```python
from build123d import *

# Parameters (mm, degrees)
SKETCH1_R             = 1.5875
SKETCH1_R_2           = 2.1844
BOSS_EXTRUDE2_DEPTH   = 1.524
BOSS_EXTRUDE3_DEPTH   = 15.875
SKETCH3_R             = 2.1844
BOSS_EXTRUDE4_DEPTH   = 1.778
BOSS_EXTRUDE4_2_DEPTH = 1.778
CUT_EXTRUDE1_DEPTH    = 9.398
SKETCH6_R             = 2.1844
BOSS_EXTRUDE5_DEPTH   = 16.256


with BuildPart() as part:
    # Sketch1 → Boss-Extrude2 (new body)
    with BuildSketch(Plane(origin=(0, 0, 0), x_dir=(1, 0, 0), z_dir=(0, 1, 0))):
        with BuildLine():
            Line((-50.746188486, 35.427401309), (-17.726188486, 35.427401309))
            ThreePointArc((-17.726188486, 35.427401309), (-16.828162874, 35.055426921), (-16.456188486, 34.157401309))
            Line((-16.456188486, 34.157401309), (-16.456188486, 27.108901309))
            ThreePointArc((-16.456188486, 27.108901309), (-16.084214098, 26.210875697), (-15.186188486, 25.838901309))
            Line((-15.186188486, 25.838901309), (-1.470188486, 25.838901309))
            ThreePointArc((-1.470188486, 25.838901309), (-0.572162874, 25.466926921), (-0.200188486, 24.568901309))
            Line((-0.200188486, 24.568901309), (-0.200188486, 10.725901309))
            ThreePointArc((-0.200188486, 10.725901309), (-0.572162874, 9.827875697), (-1.470188486, 9.455901309))
            Line((-1.470188486, 9.455901309), (-15.186188486, 9.455901309))
            ThreePointArc((-15.186188486, 9.455901309), (-16.084214098, 9.083926921), (-16.456188486, 8.185901309))
            Line((-16.456188486, 8.185901309), (-16.456188486, 1.137401309))
            ThreePointArc((-16.456188486, 1.137401309), (-16.828162874, 0.239375697), (-17.726188486, -0.132598691))
            Line((-17.726188486, -0.132598691), (-50.746188486, -0.132598691))
            ThreePointArc((-50.746188486, -0.132598691), (-51.644214098, 0.239375697), (-52.016188486, 1.137401309))
            Line((-52.016188486, 1.137401309), (-52.016188486, 34.157401309))
            ThreePointArc((-52.016188486, 34.157401309), (-51.644214098, 35.055426921), (-50.746188486, 35.427401309))
        make_face()
        with Locations(Location((-49.539688486, 32.900101309, 0), (0, 0, 90))):
            Circle(SKETCH1_R, mode=Mode.SUBTRACT)
        with Locations(Location((-18.907288486, 32.900101309, 0), (0, 0, 90))):
            Circle(SKETCH1_R, mode=Mode.SUBTRACT)
        with Locations(Location((-18.907288486, 2.394701309, 0), (0, 0, 90))):
            Circle(SKETCH1_R, mode=Mode.SUBTRACT)
        with Locations(Location((-49.539688486, 2.394701309, 0), (0, 0, 90))):
            Circle(SKETCH1_R, mode=Mode.SUBTRACT)
        with Locations(Location((-4.111788486, 21.165301309, 0), (0, 0, 90))):
            Circle(SKETCH1_R_2, mode=Mode.SUBTRACT)
        with Locations(Location((-4.111788486, 14.129501309, 0), (0, 0, 90))):
            Circle(SKETCH1_R_2, mode=Mode.SUBTRACT)
    extrude(amount=BOSS_EXTRUDE2_DEPTH)

    # Sketch2 → Boss-Extrude3 (add)
    with BuildSketch(Plane(origin=(0, 1.524, 0), x_dir=(1, 0, 0), z_dir=(0, 1, 0))):
        with BuildLine():
            Line((-0.249338446, 12.681643767), (-2.605441809, 10.307979525))
            ThreePointArc((-2.605441809, 10.307979525), (-2.77070914, 10.196884511), (-2.96598326, 10.157853612))
            Line((-2.96598326, 10.157853612), (-5.158955649, 10.157853612))
            ThreePointArc((-5.158955649, 10.157853612), (-5.354367589, 10.196941921), (-5.519707394, 10.308191511))
            Line((-5.519707394, 10.308191511), (-7.872832313, 12.681643767))
            Line((-7.872832313, 12.681643767), (-7.872832313, 24.873643767))
            ThreePointArc((-7.872832313, 24.873643767), (-7.724042558, 25.232854011), (-7.364832313, 25.381643767))
            Line((-7.364832313, 25.381643767), (-0.757338446, 25.381643767))
            ThreePointArc((-0.757338446, 25.381643767), (-0.398128202, 25.232854011), (-0.249338446, 24.873643767))
            Line((-0.249338446, 24.873643767), (-0.249338446, 12.681643767))
        make_face()
    extrude(amount=BOSS_EXTRUDE3_DEPTH)

    # Sketch4 → Cut-Extrude1 (cut)
    with BuildSketch(Plane(origin=(0, 17.399, 0), x_dir=(1, 0, 0), z_dir=(0, 1, 0))):
        Polygon((-7.237832313, 24.873643767), (-7.237832313, 12.681643767), (-5.158955649, 10.792853612), (-2.96598326, 10.792853612), (-0.884338446, 12.681643767), (-0.884338446, 24.873643767), align=None)
    extrude(amount=-CUT_EXTRUDE1_DEPTH, mode=Mode.SUBTRACT)



with BuildPart() as body_2:
    # Sketch3 → Boss-Extrude4 (new body)
    with BuildSketch(Plane.XZ):
        with Locations(Location((-4.111788486, -14.129501309, 0), (0, 0, 270))):
            Circle(SKETCH3_R)
    extrude(amount=BOSS_EXTRUDE4_DEPTH)


with BuildPart() as body_3:
    # Sketch3 → Boss-Extrude4 2 (new body)
    with BuildSketch(Plane.XZ):
        with Locations(Location((-4.111788486, -21.165301309, 0), (0, 0, 270))):
            Circle(SKETCH3_R)
    extrude(amount=BOSS_EXTRUDE4_2_DEPTH)


with BuildPart() as part_1:
    add(part.part)

    add(body_2.part)  # Boss-Extrude5 merges body 2

    add(body_3.part)  # Boss-Extrude5 merges body 3
    # Sketch6 → Boss-Extrude5 (add)
    with BuildSketch(Plane.XZ):
        with Locations(Location((-4.111788486, -14.129501309, 0), (0, 0, 90))):
            Circle(SKETCH6_R)
        with Locations(Location((-4.111788486, -21.165301309, 0), (0, 0, 270))):
            Circle(SKETCH6_R)
    extrude(amount=-BOSS_EXTRUDE5_DEPTH)


solid = part_1.part
```
Could you check a few things on this model? Use its own coordinates, in mm. A direction names the side the tool comes from. Coordinates: 2 decimals unless noted, no trailing zeros. Write each loop counter-clockwise with the first axis right and the second up, starting at its lowest first coordinate (ties: lowest second). Pieces come first, ordered by that corner, then holes. Notation, with made-up numbers: (19.25, -9) -> (71.25, -9) arc R17 ccw to (71.25, 11) -> close; hole circle Ø4 at (4.25, -8.75). An arc over 180 degrees is marked (long way). One line per question, with ' | ' between items. Start each with the question number.
1. If we section it at C-C (y = 3.5): Please give me the cut outline in (x, z), and give its area (3 significant figures).
2. For faces 5 (the face through (-1.41, 9.35, -11.51)), 6 (the face through (-16.456, 1, -31)), 7 (the face through (-5.4, -0.9, -19.4)), 8 (the face through (-0.249, 9, -19)), 9 (the face through (-4, 16.256, -14)), which set-ups out of +Z, -Z, +X, -X, +Y, -Y let a thin tool reach every point of the face, with its end or its side?
3. Please list where these lines run through material, in increasing order: line 1 along X through (y, z) = (9, -14); line 2 along X through (y, z) = (8.5, -24); line 3 along X through (y, z) = (14, -16).
4. Will these pins go through, and if not, where does the flat tip stop? P1, Ø1.7, axis at x = -6.5, y = 0.5, coming from the +Z side; P2, Ø12, axis at x = -13, z = -26, coming from the -Y side; P3, Ø10, axis at x = -42, z = -27.5, coming from the +Y side.
5. If we section it at D-D (x = -25): Please give me the cut outline in (y, z).
6. Thinking about a two-plate mould opening in Z: for faces 1 (the face through (-4, 9, -25.382)), 2 (the face through (-4, 13, -24.874)), 3 (the face through (-4, -1.778, -21)), 4 (the face through (-50.61, 0.75, -1.22)), which applies, pulls with the +Z half, pulls with the -Z half, needs draft (parallel to the pull), parting line crosses it, or undercut?
7. If we section it at B-B (y = 11.25): Please give me the cut outline in (x, z), and give its area (3 significant figures).
8. If we section it at A-A (z = -17.5): Please give me the cut outline in (x, y).
Return value:
1) outline: (-7.87, -24.87) arc R0.51 ccw to (-7.36, -25.38) -> (-0.76, -25.38) arc R0.51 ccw to (-0.25, -24.87) -> (-0.25, -12.68) -> (-2.61, -10.31) arc R0.51 ccw to (-2.97, -10.16) -> (-5.16, -10.16) arc R0.51 ccw to (-5.52, -10.31) -> (-7.87, -12.68) -> close | area: 110 mm²
2) face 5: +Z, +X, +Y | face 6: -Z, +X, +Y, -Y | face 7: -Y | face 8: +Z, -Z, +X, +Y | face 9: +Y
3) line 1: x = -7.87 to -7.24, -6.29 to -1.93, -0.88 to -0.25 | line 2: x = -7.87 to -7.24, -0.88 to -0.25 | line 3: x = -7.87 to -7.24, -5.24 to -2.98, -0.88 to -0.25
4) P1: stops at z = -9.46 | P2: stops at y = 0 | P3: stops at y = 1.52
5) outline: (0, -35.43) -> (1.52, -35.43) -> (1.52, 0.13) -> (0, 0.13) -> close
6) face 1: pulls with the -Z half | face 2: undercut | face 3: needs draft | face 4: undercut
7) outline: (-7.87, -24.87) arc R0.51 ccw to (-7.36, -25.38) -> (-0.76, -25.38) arc R0.51 ccw to (-0.25, -24.87) -> (-0.25, -12.68) -> (-2.61, -10.31) arc R0.51 ccw to (-2.97, -10.16) -> (-5.16, -10.16) arc R0.51 ccw to (-5.52, -10.31) -> (-7.87, -12.68) -> close; circle Ø4.37 at (-4.11, -21.17); circle Ø4.37 at (-4.11, -14.13); hole (-7.24, -24.87) -> (-0.88, -24.87) -> (-0.88, -12.68) -> (-2.97, -10.79) -> (-5.16, -10.79) -> (-7.24, -12.68) -> close | area: 54.1 mm²
8) outline: (-52.02, 0) -> (-0.2, 0) -> (-0.2, 1.52) -> (-0.25, 1.52) -> (-0.25, 17.4) -> (-0.88, 17.4) -> (-0.88, 8) -> (-7.24, 8) -> (-7.24, 17.4) -> (-7.87, 17.4) -> (-7.87, 1.52) -> (-52.02, 1.52) -> close
